Work out the finished part from the listing and answer in its coordinate system (mm). A direction names the side the tool comes from. Give positions to 0.01 mm unless a question says otherwise; leave off trailing zeros. Loops run counter-clockwise (first coordinate to the right, second up) from the corner with the lowest first, then second, coordinate; pieces in that order, holes last. Notation, with made-up numbers: M 75,-33 L 86,-33 A11 cw 86,-20 Z; hole C 4.5,7.25 d2. An arc over 180 degrees is marked long. Write item = value, one per line. Start each with the question number.
1. Section A-A on y = -3.75 is taken. Determine the outline of the cut face in (x, z), plus the area to 3 significant figures.
2. Section C-C on x = 94 is taken. Determine the outline of the cut face in (y, z).
3. Consider L1, parallel to Z at x = 90.5, y = -4.5. Determine where the line is inside the solid, lowest interval first. Write a range as [from, to].
4. The mould has two halves that part along Y. Classify faces 1 (the face through (108, 7.5, 0)), 2 (the face through (108, 6.5, 0)), 3 (the face through (108, 0, 7.5)): released by +Y, released by -Y, zero draft, split by the parting line, or undercut.
5. For faces 4 (the face through (108, 0, 6.5)), 5 (the face through (0, 0, 7)), determine the directions among +Z, -Z, +X, -X, +Y, -Y from which every point of the face is accessible in a straight line to the end or side of a thin tool.
```python
from build123d import *

# Parameters (mm, degrees)
SKETCH_1_W          = 15
SKETCH_1_H          = 15
SKETCH_1_W_2        = 13
SKETCH_1_H_2        = 13
EXTRUDE_1_DEPTH     = 220
SKETCH_2_R          = 1.45
SKETCH_2_R_2        = 1.6
CUT_EXTRUDE_1_DEPTH = 221.638278637


with BuildPart() as part:
    # 草图1 → 凸台-拉伸1 (new body)
    with BuildSketch(Plane(origin=(0, 0, 0), x_dir=(0, 0, -1), z_dir=(1, 0, 0))):
        Rectangle(SKETCH_1_W, SKETCH_1_H)
        Rectangle(SKETCH_1_W_2, SKETCH_1_H_2, mode=Mode.SUBTRACT)
    extrude(amount=EXTRUDE_1_DEPTH)

    # 草图2 → 切除-拉伸1 (cut, through all)
    with BuildSketch(Plane.XY.offset(7.5)):
        with Locations((215, 0)):
            Circle(SKETCH_2_R)
        with Locations((205, 0)):
            Circle(SKETCH_2_R)
        with Locations((123.545188216, 0)):
            Circle(SKETCH_2_R_2)
        with Locations((113.545188216, 0)):
            Circle(SKETCH_2_R_2)
        with Locations((103.545188216, 0)):
            Circle(SKETCH_2_R_2)
        with Locations((15, 0)):
            Circle(SKETCH_2_R)
        with Locations((5, 0)):
            Circle(SKETCH_2_R)
    extrude(amount=-CUT_EXTRUDE_1_DEPTH, mode=Mode.SUBTRACT)


solid = part.part
```
Verdict:
q1.outline = M 0,-7.5 L 220,-7.5 L 220,-6.5 L 0,-6.5 Z; M 0,6.5 L 220,6.5 L 220,7.5 L 0,7.5 Z
q1.area = 440 mm2
q2.outline = M -7.5,-7.5 L 7.5,-7.5 L 7.5,7.5 L -7.5,7.5 Z; hole M -6.5,-6.5 L 6.5,-6.5 L 6.5,6.5 L -6.5,6.5 Z
q3.L1 = [-7.5, -6.5], [6.5, 7.5]
q4.face_1 = released by +Y
q4.face_2 = undercut
q4.face_3 = zero draft
q5.face_4 = +X, -X
q5.face_5 = +Z, -Z, -X, +Y, -Y
